from build123d import *

# Parameters (mm, degrees)
SKETCH_1_R           = 19
SKETCH_1_R_2         = 17
EXTRUDE_1_DEPTH      = 30
SKETCH_16_R          = 17
EXTRUDE_9_DEPTH      = 3
SKETCH_4_R           = 9
EXTRUDE_2_DEPTH      = 10
CUT_EXTRUDE_8_DEPTH  = 10
EXTRUDE_10_DEPTH     = 30
SKETCH_6_R           = 2.25
CUT_EXTRUDE_9_DEPTH  = 70
SKETCH_9_R           = 21
SKETCH_9_R_2         = 19
EXTRUDE_4_DEPTH      = 2
SKETCH_10_R          = 21
SKETCH_10_R_2        = 19
EXTRUDE_5_DEPTH      = 2
EXTRUDE_START        = -2
SKETCH_11_R          = 21
SKETCH_11_R_2        = 19
EXTRUDE_6_DEPTH      = 2
EXTRUDE_START_2      = 2
SKETCH_12_R          = 21
SKETCH_12_R_2        = 19
EXTRUDE_7_DEPTH      = 2
SKETCH_13_W          = 6
SKETCH_13_H          = 6
CUT_EXTRUDE_5_DEPTH  = 2
SKETCH_14_R          = 2.15
EXTRUDE_11_DEPTH     = 5
SKETCH_22_R          = 6.15
CUT_EXTRUDE_10_DEPTH = 4
SKETCH_25_R          = 4.5
CUT_EXTRUDE_11_DEPTH = 2


with BuildPart() as part:
    # Sketch 1 → Extrude 1 (new body)
    with BuildSketch(Plane.XY):
        Circle(SKETCH_1_R)
        Circle(SKETCH_1_R_2, mode=Mode.SUBTRACT)
    extrude(amount=EXTRUDE_1_DEPTH)



with BuildPart() as body_2:
    # Sketch 16 → Extrude 9 (new body)
    with BuildSketch(Plane(origin=(0, 0, 0), x_dir=(-1, 0, 0), z_dir=(0, 0, -1))):
        with Locations(Location((0, 0, 0), (0, 0, 180))):
            Circle(SKETCH_16_R)
    extrude(amount=EXTRUDE_9_DEPTH)

    # Sketch 7 → Cut-Extrude 8 (cut)
    with BuildSketch(Plane(origin=(0, 0, -3), x_dir=(-1, 0, 0), z_dir=(0, 0, -1))):
        with BuildLine():
            Line((-8.304923146, 14.833349303), (-3.539760668, 8.274665819))
            ThreePointArc((-3.539760668, 8.274665819), (0, 9), (3.539760668, 8.274665819))
            Line((3.539760668, 8.274665819), (8.304923146, 14.833349303))
            ThreePointArc((8.304923146, 14.833349303), (0, 17), (-8.304923146, 14.833349303))
        make_face()
        with BuildLine():
            ThreePointArc((9, 0), (8.990875637, -0.405160803), (8.96352105, -0.809500088))
            Line((8.96352105, -0.809500088), (16.673715902, -3.314694257))
            ThreePointArc((16.673715902, -3.314694257), (16.91823233, -1.665357269), (17, 0))
            ThreePointArc((17, 0), (15.575571404, 6.811870187), (11.540991124, 12.482208294))
            Line((11.540991124, 12.482208294), (6.775828645, 5.92352481))
            ThreePointArc((6.775828645, 5.92352481), (8.425629288, 3.163664188), (9, 0))
        make_face()
        with BuildLine():
            ThreePointArc((7.727453072, -4.613726153), (5.290067271, -7.281152949), (2, -8.774964387))
            Line((2, -8.774964387), (2, -16.881943016))
            ThreePointArc((2, -16.881943016), (9.992349289, -13.753288904), (15.437647924, -7.118920323))
            Line((15.437647924, -7.118920323), (7.727453072, -4.613726153))
        make_face()
        with BuildLine():
            Line((-2, -16.881943016), (-2, -8.774964387))
            ThreePointArc((-2, -8.774964387), (-5.290067271, -7.281152949), (-7.727453072, -4.613726153))
            Line((-7.727453072, -4.613726153), (-15.437647924, -7.118920323))
            ThreePointArc((-15.437647924, -7.118920323), (-9.992349289, -13.753288904), (-2, -16.881943016))
        make_face()
        with BuildLine():
            Line((-16.673715902, -3.314694257), (-8.96352105, -0.809500088))
            ThreePointArc((-8.96352105, -0.809500088), (-8.559508647, 2.781152949), (-6.775828645, 5.92352481))
            Line((-6.775828645, 5.92352481), (-11.540991124, 12.482208294))
            ThreePointArc((-11.540991124, 12.482208294), (-16.167960777, 5.253288904), (-16.673715902, -3.314694257))
        make_face()
    extrude(amount=-CUT_EXTRUDE_8_DEPTH, mode=Mode.SUBTRACT)


with BuildPart() as body_3:
    # Sketch 4 → Extrude 2 (new body)
    with BuildSketch(Plane.XY):
        Circle(SKETCH_4_R)
    extrude(amount=EXTRUDE_2_DEPTH)


with BuildPart() as part_1:
    add(part.part)

    add(body_2.part)  # Extrude 10 merges body 2

    add(body_3.part)  # Extrude 10 merges body 3
    # Sketch 21 → Extrude 10 (add)
    with BuildSketch(Plane.XY):
        with BuildLine():
            ThreePointArc((-6.775828645, 5.92352481), (-5.290067271, 7.281152949), (-3.539760668, 8.274665819))
            Line((-3.539760668, 8.274665819), (-8.304923146, 14.833349303))
            ThreePointArc((-8.304923146, 14.833349303), (-9.992349289, 13.753288904), (-11.540991124, 12.482208294))
            Line((-11.540991124, 12.482208294), (-6.775828645, 5.92352481))
        make_face()
        with BuildLine():
            Line((8.304923146, 14.833349303), (3.539760668, 8.274665819))
            ThreePointArc((3.539760668, 8.274665819), (5.290067271, 7.281152949), (6.775828645, 5.92352481))
            Line((6.775828645, 5.92352481), (11.540991124, 12.482208294))
            ThreePointArc((11.540991124, 12.482208294), (9.992349289, 13.753288904), (8.304923146, 14.833349303))
        make_face()
        with BuildLine():
            Line((16.673715902, -3.314694257), (8.96352105, -0.809500088))
            ThreePointArc((8.96352105, -0.809500088), (8.559508647, -2.781152949), (7.727453072, -4.613726153))
            Line((7.727453072, -4.613726153), (15.437647924, -7.118920323))
            ThreePointArc((15.437647924, -7.118920323), (16.167960777, -5.253288904), (16.673715902, -3.314694257))
        make_face()
        with BuildLine():
            Line((2, -16.881943016), (2, -8.774964387))
            ThreePointArc((2, -8.774964387), (0, -9), (-2, -8.774964387))
            Line((-2, -8.774964387), (-2, -16.881943016))
            ThreePointArc((-2, -16.881943016), (0, -17), (2, -16.881943016))
        make_face()
        with BuildLine():
            ThreePointArc((-7.727453072, -4.613726153), (-8.559508647, -2.781152949), (-8.96352105, -0.809500088))
            Line((-8.96352105, -0.809500088), (-16.673715902, -3.314694257))
            ThreePointArc((-16.673715902, -3.314694257), (-16.167960777, -5.253288904), (-15.437647924, -7.118920323))
            Line((-15.437647924, -7.118920323), (-7.727453072, -4.613726153))
        make_face()
    extrude(amount=EXTRUDE_10_DEPTH)

    # Sketch 6 → Cut-Extrude 9 (cut)
    with BuildSketch(Plane.XY.offset(-3)):
        Circle(SKETCH_6_R)
    extrude(amount=CUT_EXTRUDE_9_DEPTH, mode=Mode.SUBTRACT)

    # Sketch 9 → Extrude 4 (add)
    with BuildSketch(Plane.XY):
        Circle(SKETCH_9_R)
        Circle(SKETCH_9_R_2, mode=Mode.SUBTRACT)
    extrude(amount=EXTRUDE_4_DEPTH)

    # Sketch 10 → Extrude 5 (add)
    with BuildSketch(Plane.XY.offset(6)):
        Circle(SKETCH_10_R)
        Circle(SKETCH_10_R_2, mode=Mode.SUBTRACT)
    extrude(amount=EXTRUDE_5_DEPTH)

    # Sketch 11 → Extrude 6 (add)
    with BuildSketch(Plane.XY.offset(30).offset(EXTRUDE_START)):
        Circle(SKETCH_11_R)
        Circle(SKETCH_11_R_2, mode=Mode.SUBTRACT)
    extrude(amount=EXTRUDE_6_DEPTH)

    # Sketch 12 → Extrude 7 (add)
    with BuildSketch(Plane(origin=(0, 0, 24), x_dir=(-1, 0, 0), z_dir=(0, 0, -1)).offset(EXTRUDE_START_2)):
        with Locations(Location((0, 0, 0), (0, 0, 180))):
            Circle(SKETCH_12_R)
        Circle(SKETCH_12_R_2, mode=Mode.SUBTRACT)
    extrude(amount=-EXTRUDE_7_DEPTH)

    # Sketch 13 → Cut-Extrude 5 (cut)
    with BuildSketch(Plane.XY.offset(10)):
        Rectangle(SKETCH_13_W, SKETCH_13_H)
    extrude(amount=-CUT_EXTRUDE_5_DEPTH, mode=Mode.SUBTRACT)

    # Sketch 14 → Extrude 11 (add)
    with BuildSketch(Plane(origin=(0, 0, -3), x_dir=(-1, 0, 0), z_dir=(0, 0, -1))):
        Polygon((-11.1, -6.408587988), (0, -12.817175976), (11.1, -6.408587988), (11.1, 6.408587988), (0, 12.817175976), (-11.1, 6.408587988), align=None)
        Circle(SKETCH_14_R, mode=Mode.SUBTRACT)
    extrude(amount=EXTRUDE_11_DEPTH)

    # Sketch 22 → Cut-Extrude 10 (cut)
    with BuildSketch(Plane(origin=(0, 0, -8), x_dir=(-1, 0, 0), z_dir=(0, 0, -1))):
        Circle(SKETCH_22_R)
    extrude(amount=-CUT_EXTRUDE_10_DEPTH, mode=Mode.SUBTRACT)

    # Sketch 25 → Cut-Extrude 11 (cut)
    with BuildSketch(Plane(origin=(0, 0, -4), x_dir=(-1, 0, 0), z_dir=(0, 0, -1))):
        Circle(SKETCH_25_R)
    extrude(amount=-CUT_EXTRUDE_11_DEPTH, mode=Mode.SUBTRACT)

    # Sketch 28 → Cut-Revolve 1 (revolve, cut)
    with BuildSketch(Plane(origin=(0, 0, 0), x_dir=(0.9510565162951539, -0.3090169943749465, 0), z_dir=(-0.3090169943749465, -0.9510565162951539, 0)), mode=Mode.PRIVATE) as cut_revolve_1_sk:
        Polygon((17, 30), (9, 10), (9, 30), align=None)
    revolve(cut_revolve_1_sk.sketch.rotate(Axis((0, 0, 0), (0, 0, 1)), 198), axis=Axis((0, 0, 0), (0, 0, 1)), mode=Mode.SUBTRACT)


solid = part_1.part
Input: part model. Units: mm. Frame: model coordinates. A direction names the side the tool comes from. Coordinates: 2 decimals unless noted, no trailing zeros. Loops run counter-clockwise (first coordinate to the right, second up) from the corner with the lowest first, then second, coordinate; pieces in that order, holes last. Notation, with made-up numbers: (55.25, 38.5) - (96.25, 38.5) arc R37 cw to (96.25, 76.5) - close; hole circle Ø6 at (10.5, 49). An arc over 180 degrees is marked (long way). Answer in a Markdown table with one row per item. Add a question column.
Item 1: Section query C-C on y = 11. State how many separate pieces and enclosed holes the cut face has, then the cut area to 3 significant figures.
Item 2: Line query: line 1 along Y through (x, z) = (0, 1); line 2 along Z through (x, y) = (4, 19); line 3 along Y through (x, z) = (0, 4). Output: solid intervals per line, ascending. Write a range as [from, to].
Item 3: Section query B-B on z = 15. Return the cut outline in (x, y).
Item 4: Mould query, pull axis Y, two halves, no side actions, for faces 4 (the flat face through (5.47, 9.66, -5.46)), 5 (the flat face through (-16, -11, 8)), 6 (the cylindrical face through (16.205, 5.138, 14.79)). Classes: released by +Y, released by -Y, zero draft, split by the parting line, or undercut.
Item 5: Contact query for flat-ended pins moving along their axis: P1, Ø6, axis at y = -14, z = 5, coming from the +X side; P2, Ø3.5, axis at x = -5.5, y = -8, coming from the +Z side; P3, Ø3, axis at x = -6.5, z = 2, coming from the +Y side; P4, Ø10, axis at x = -1, y = -2, coming from the -Z side. Output: stop coordinate, or through.
Item 6: Section query A-A on z = 9. Return the cut outline in (x, y), then the cut area to 3 significant figures.
Item 7: Access query for faces 1 (the flat face through (0, -3, 9)), 2 (the cylindrical face through (0, -17, -1)), 3 (the flat face through (-16, 11, 22)). Directions: +Z, -Z, +X, -X, +Y, -Y. A direction counts if a zero-diameter tool reaches every point of the face in a straight line with its end or side. Return the directions, or none.
Recorded:
| question | item | result |
|---|---|---|
| 1 | separate pieces | 5 |
| 1 | enclosed holes | 0 |
| 1 | area | 465 mm^2 |
| 2 | line 1 | [-21, -2.25], [2.25, 9], [17, 21] |
| 2 | line 2 | [0, 2], [6, 8], [22, 24], [28, 30] |
| 2 | line 3 | [-19, -2.25], [2.25, 9], [17, 19] |
| 3 | outline | circle Ø38 at (0, 0); hole (-16.67, -3.31) - (-10.91, -1.44) arc R11 ccw to (-9.67, -5.24) - (-15.44, -7.12) arc R17 ccw to (-2, -16.88) - (-2, -10.82) arc R11 ccw to (2, -10.82) - (2, -16.88) arc R17 ccw to (15.44, -7.12) - (9.67, -5.24) arc R11 ccw to (10.91, -1.44) - (16.67, -3.31) arc R17 ccw to (11.54, 12.48) - (7.98, 7.58) arc R11 ccw to (4.74, 9.93) - (8.3, 14.83) arc R17 ccw to (-8.3, 14.83) - (-4.74, 9.93) arc R11 ccw to (-7.98, 7.58) - (-11.54, 12.48) arc R17 ccw to start |
| 4 | face 4 | released by +Y |
| 4 | face 5 | zero draft |
| 4 | face 6 | undercut |
| 5 | P1 | x = 17.78 |
| 5 | P2 | z = 10 |
| 5 | P3 | y = 20.4 |
| 5 | P4 | z = -8 |
| 6 | outline | circle Ø38 at (0, 0); hole (-16.67, -3.31) - (-8.96, -0.81) arc R9 cw to (-6.78, 5.92) - (-11.54, 12.48) arc R17 ccw to start; hole (-15.44, -7.12) arc R17 ccw to (-2, -16.88) - (-2, -8.77) arc R9 cw to (-7.73, -4.61) - close; hole (-8.3, 14.83) - (-3.54, 8.27) arc R9 cw to (3.54, 8.27) - (8.3, 14.83) arc R17 ccw to start; hole (-3, -3) - (3, -3) - (3, 3) - (-3, 3) - close; hole (2, -16.88) arc R17 ccw to (15.44, -7.12) - (7.73, -4.61) arc R9 cw to (2, -8.77) - close; hole (6.78, 5.92) arc R9 cw to (8.96, -0.81) - (16.67, -3.31) arc R17 ccw to (11.54, 12.48) - close |
| 6 | area | 605 mm^2 |
| 7 | face 1 | +Z |
| 7 | face 2 | -Z, -Y |
| 7 | face 3 | none |
